Here's how the part is built. I have some questions about the finished solid (model axes, mm). Face numbers are marked on the shaded views. A direction names the side the tool comes from. Round coordinates to 2 decimals unless told otherwise and drop trailing zeros.
```python
from build123d import *

# Parameters (mm, degrees)
ESBO_O3_R             = 2
CORTE_EXTRUS_O1_DEPTH = 8
PADR_OCIRCULAR1_COUNT = 8
FILETE2_R             = 0.25


with BuildPart() as part:
    # Esbo_o2 → Revolu_o1 (revolve)
    with BuildSketch(Plane(origin=(0, 0, 0), x_dir=(1, 0, 0), z_dir=(0, 1, 0)), mode=Mode.PRIVATE) as revolu_o1_sk:
        Polygon((0, 0), (-13.75, 0), (-13.75, 2.2), (-11.75, 2.2), (-11.75, 5), (-13.75, 5), (-13.75, 13), (-11.75, 13), (0, 13), align=None)
    revolve(revolu_o1_sk.sketch.rotate(Axis((0, 0, 0), (0, 0, -1)), 180), axis=Axis((0, 0, 0), (0, 0, -1)))

    # Esbo_o3 → Corte-extrus_o1 (cut)
    with BuildSketch(Plane(origin=(0, 13.75, 0), x_dir=(1, 0, 0), z_dir=(0, 1, 0))):
        with Locations(Location((0, 9, 0), (0, 0, 270))):
            Circle(ESBO_O3_R)
    corte_extrus_o1 = extrude(amount=-CORTE_EXTRUS_O1_DEPTH, mode=Mode.SUBTRACT)

    # Padr_oCircular1: Corte-extrus_o1 ×8 about axis
    padr_ocircular1_axis = Axis((0, 0, 0), (0, 0, 1))
    for i in range(1, PADR_OCIRCULAR1_COUNT):
        add(corte_extrus_o1.rotate(padr_ocircular1_axis, i * 360 / PADR_OCIRCULAR1_COUNT), mode=Mode.SUBTRACT)

    # Esbo_o12 → Corte-Revolu_o1 (revolve, cut)
    with BuildSketch(Plane(origin=(0, 0, 0), x_dir=(1, 0, 0), z_dir=(0, 1, 0)), mode=Mode.PRIVATE) as corte_revolu_o1_sk:
        Polygon((-4, 7.75), (-11.75, 0), (-2.977226814, 0), (0, 0), (0, 13), (-2.977226814, 13), (-5.91084373, 13), align=None)
    revolve(corte_revolu_o1_sk.sketch.rotate(Axis((0, 0, 0), (0, 0, -1)), 180), axis=Axis((0, 0, 0), (0, 0, -1)), mode=Mode.SUBTRACT)

    # Filete2
    filete2_edges = [part.edges().sort_by_distance(p)[0] for p in [
        (-4, 0, -7.75),
    ]]
    fillet(filete2_edges, radius=FILETE2_R)


solid = part.part
```
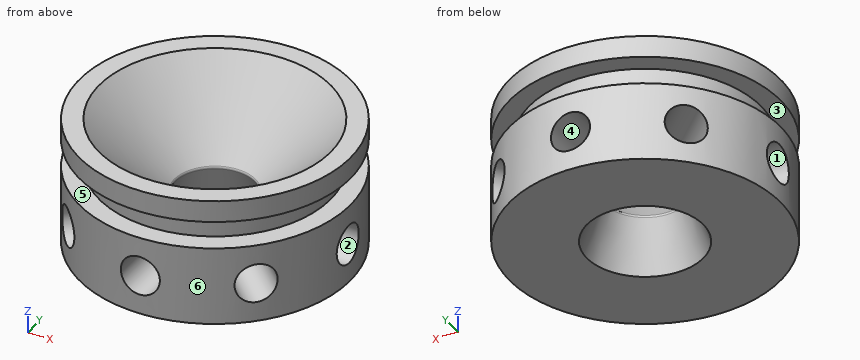
1) I'm going to push flat-ended pins straight in: pin 1 (14 mm diameter, centred on x = 4, y = 2.5, fed in from +Z); pin 2 (3 mm diameter, centred on y = 0, z = -9, fed in from -X); pin 3 (4 mm diameter, centred on y = -2.5, z = -6, fed in from +X); pin 4 (3 mm diameter, centred on x = 0, z = -10, fed in from -Y). Where does each tip first touch, or does it pass through?
2) If we section it at B-B (y = 3): Give the number of separate pieces and of enclosed holes in the cut face, plus the area to 3 significant figures.
3) For the marked faces 1, 2 and 3, which set-ups out of +Z, -Z, +X, -X, +Y, -Y let a thin tool reach every point of the face, with its end or its side?
4) I need wall thicknesses on line 1 (Z direction, x = 9.75, y = -9.5); line 2 (Y direction, x = -5.25, z = -10); line 3 (Y direction, x = 7.75, z = -9). Which ranges of each line are inside material? Lowest first, please.
5) We'd pull the mould along X, two halves only. Please class the marked faces 4, 5 and 6: +X half, -X half, draft (parallel to the pull), parting line (faces both ways), or undercut.
Solutions:
1. pin 1: stops at z = -0.03
1. pin 2: stops at x = -5.75
1. pin 3: stops at x = 13.74
1. pin 4: stops at y = -13.75
2. separate pieces: 2
2. enclosed holes: 2
2. area: 182 mm2
3. face 1: -X
3. face 2: +X
3. face 3: none
4. line 1: z = -13 to -10.99, -7.01 to -5, -2.2 to 0
4. line 2: y = -12.71 to -7.7, -2.88 to 2.88, 7.7 to 12.71
4. line 3: y = -11.36 to -10.58, -4.92 to -2, 2 to 4.92, 10.58 to 11.36
5. face 4: undercut
5. face 5: draft
5. face 6: parting line
